The model under review builds one solid part; all positions refer to its coordinate system, in mm. A direction names the side the tool comes from. Round coordinates to 2 decimals unless told otherwise and drop trailing zeros. Loops run counter-clockwise (first coordinate to the right, second up) from the corner with the lowest first, then second, coordinate; pieces in that order, holes last. Notation, with made-up numbers: M 1,-30.75 L 48,-30.75 A29 cw 48,-5.75 Z; hole C 36,-33 d5. An arc over 180 degrees is marked long. Return JSON: item names as keys, results as strings. Group by question number.
Q1. For faces 1 (the face through (78, 17, 0.5)), 2 (the face through (78, 3, 0.5)), 3 (the face through (78, 108, 0.5)), 4 (the face through (78, 74, 1)), 5 (the face through (78, 60, 0)), list the 3-axis set-ups (+Z, -Z, +X, -X, +Y, -Y) from which the entire face can be reached by the end or side of a thin tool; tool diameter is ignored.
Q2. Consider section A-A (x = 149). State the section outline as (y, z) points, and give its area (3 significant figures).
Q3. To check wall thickness, follow line 1 along Y through (x, z) = (9.5, 0.65); line 2 along Z through (x, y) = (30.5, 33). State the ranges of each line that lie inside material, in increasing order.
Q4. Clearance check with flat-ended pins moving along their axes: pin 1 Ø0.6 at (x, z) = (98.5, 0.5) entering from -Y; pin 2 Ø0.6 at (x, z) = (60.5, 1) entering from -Y; pin 3 Ø3 at (x, y) = (41.5, 81.5) entering from +Z; pin 4 Ø0.6 at (x, z) = (105, 1) entering from +Y. State where each tip first meets the part, or that it passes through.
Q5. Draft analysis for pull direction Y (two halves, no side actions). For faces 6 (the face through (78, 66, 0.5)), 7 (the face through (78, 58, 1)), state which applies: pulls with the +Y half, pulls with the -Y half, needs draft (parallel to the pull), parting line crosses it, or undercut.
Q6. Consider section B-B (z = 0.8). State the section outline as (x, y) points, and give its area (3 significant figures).
Q7. Consider section C-C (y = 79.5). State the section outline as (x, z) points, and give its area (4 significant figures).
Autodesk Inventor part; units mm, degrees
ref_plane "YZ Plane" through (0, 0, 0) normal (1, 0, 0) x (0, 1, 0)
ref_plane "XZ Plane" through (0, 0, 0) normal (0, 1, 0) x (-1, 0, 0)
ref_plane "XY Plane" through (0, 0, 0) normal (0, 0, 1) x (1, 0, 0)
sketch "Эскиз3" plane through (0, 0, 0) normal (0, 0, 1) x (1, 0, 0)
  line L0 (0, 0) -> (158.5, 0)
  line L1 (158.5, 0) -> (158.5, 117.5)
  line L2 (158.5, 117.5) -> (0, 117.5)
  line L3 (0, 117.5) -> (0, 0)
  dimension "d25" = 117.5
  dimension "d26" = 158.5
extrude "Выдавливание2" add sketch "Эскиз3" along normal blind 1
sketch "Эскиз4" plane through (0, 0, 1) normal (0, 0, 1) x (1, 0, 0)
  line L0 (158.5, 117.5) -> (0, 117.5)
  line L1 (0, 117.5) -> (158.5, 117.5)
  line L2 (158.5, 117.5) -> (158.5, 97.5)
  line L3 (158.5, 97.5) -> (0, 97.5)
  line L4 (0, 97.5) -> (0, 117.5)
  line L5 (0, 117.5) -> (0, 0)
  line L6 (0, 87.75) -> (158.5, 87.75)
  line L7 (158.5, 87.75) -> (158.5, 77.25)
  line L8 (158.5, 77.25) -> (0, 77.25)
  line L9 (0, 77.25) -> (0, 87.75)
  line L10 (0, 71.25) -> (158.5, 71.25)
  line L11 (0, 60.75) -> (158.5, 60.75)
  line L12 (0, 54.75) -> (158.5, 54.75)
  line L13 (0, 44.25) -> (158.5, 44.25)
  line L14 (0, 38.25) -> (158.5, 38.25)
  line L15 (0, 27.75) -> (158.5, 27.75)
  line L16 (0, 21.75) -> (158.5, 21.75)
  line L17 (0, 11.25) -> (158.5, 11.25)
  line L18 (0, 5.25) -> (158.5, 5.25)
  line L19 (0, 0) -> (158.5, 0)
  line L20 (0, 0) -> (158.5, 0)
  line L21 (0, 71.25) -> (0, 60.75)
  line L22 (0, 54.75) -> (0, 44.25)
  line L23 (0, 38.25) -> (0, 27.75)
  line L24 (0, 21.75) -> (0, 11.25)
  line L25 (0, 5.25) -> (0, 0)
  line L26 (158.5, 0) -> (158.5, 5.25)
  line L27 (158.5, 11.25) -> (158.5, 21.75)
  line L28 (158.5, 27.75) -> (158.5, 38.25)
  line L29 (158.5, 44.25) -> (158.5, 54.75)
  line L30 (158.5, 0) -> (158.5, 117.5)
  line L31 (158.5, 60.75) -> (158.5, 71.25)
  dimension "d29" = 20
  dimension "d30" = 9.75
  dimension "d31" = 10.5
  dimension "d32" = 6
  dimension "d35" = 10.5
  dimension "d36" = 6
  dimension "d37" = 10.5
  dimension "d38" = 6
  dimension "d39" = 10.5
  dimension "d40" = 6
  dimension "d41" = 10.5
  dimension "d42" = 6
  dimension "d43" = 5.25
extrude "Выдавливание3" cut sketch "Эскиз4" against normal blind 0.5 contours L2 L3 L4 L0 | L7 L8 L5 L6 | L30 L11 L5 L10 | L29 L13 L5 L12 | L28 L15 L5 L14 | L27 L17 L5 L16 | L26 L19 L5 L18
properties part number "Подложка"
Values:
{
 "1": {"face 1": "+Z, +X, -X", "face 2": "+Z, +X, -X, -Y", "face 3": "+Z, +X, -X, +Y", "face 4": "+Z, +X, -X, +Y, -Y", "face 5": "-Z, +X, -X, +Y, -Y"},
 "2": {"outline": "M 0,0 L 117.5,0 L 117.5,0.5 L 97.5,0.5 L 97.5,1 L 87.75,1 L 87.75,0.5 L 77.25,0.5 L 77.25,1 L 71.25,1 L 71.25,0.5 L 60.75,0.5 L 60.75,1 L 54.75,1 L 54.75,0.5 L 44.25,0.5 L 44.25,1 L 38.25,1 L 38.25,0.5 L 27.75,0.5 L 27.75,1 L 21.75,1 L 21.75,0.5 L 11.25,0.5 L 11.25,1 L 5.25,1 L 5.25,0.5 L 0,0.5 Z", "area": "78.6 mm2"},
 "3": {"line 1": "y = 5.25 to 11.25, 21.75 to 27.75, 38.25 to 44.25, 54.75 to 60.75, 71.25 to 77.25, 87.75 to 97.5", "line 2": "z = 0 to 0.5"},
 "4": {"pin 1": "stops at y = 0", "pin 2": "stops at y = 5.25", "pin 3": "stops at z = 0.5", "pin 4": "stops at y = 97.5"},
 "5": {"face 6": "undercut", "face 7": "needs draft"},
 "6": {"outline": "M 0,5.25 L 158.5,5.25 L 158.5,11.25 L 0,11.25 Z; M 0,21.75 L 158.5,21.75 L 158.5,27.75 L 0,27.75 Z; M 0,38.25 L 158.5,38.25 L 158.5,44.25 L 0,44.25 Z; M 0,54.75 L 158.5,54.75 L 158.5,60.75 L 0,60.75 Z; M 0,71.25 L 158.5,71.25 L 158.5,77.25 L 0,77.25 Z; M 0,87.75 L 158.5,87.75 L 158.5,97.5 L 0,97.5 Z", "area": "6,300 mm2"},
 "7": {"outline": "M 0,0 L 158.5,0 L 158.5,0.5 L 0,0.5 Z", "area": "79.25 mm2"}
}
